Verification items for the finished model (mm, model axes). Round coordinates to 2 decimals unless told otherwise and drop trailing zeros. Write each loop counter-clockwise with the first axis right and the second up, starting at its lowest first coordinate (ties: lowest second). Pieces come first, ordered by that corner, then holes. Notation, with made-up numbers: M -3,8 L 54,8 A17 ccw 54,33 Z; hole C 26.5,22.5 d7. An arc over 180 degrees is marked long. One line per item, written item: value. Start each with the question number.
Item 1: Section check B-B, the plane x = -10. Record the cut outline in (y, z), then the cut area to 3 significant figures.
Item 2: Gauge pin test, flat ends, axial feed: pin 1 (4.5 mm diameter, centred on y = 0, z = 7.5, fed in from -X); pin 2 (12 mm diameter, centred on y = -8, z = 19, fed in from +X); pin 3 (10 mm diameter, centred on x = 9.5, z = 19, fed in from -Y); pin 4 (1 mm diameter, centred on x = 5, z = 7, fed in from +Y). Record the tip position at first contact, or that the pin passes through.
Item 3: Section check A-A, the plane y = 0. Record the cut outline in (x, z), then the cut area to 4 significant figures.
Item 4: Thickness scan on probe 1 along X at (y, z) = (0, 3); probe 2 along Y at (x, z) = (-9, 7). Record the ranges inside material, lowest first. Write a range as from..to.
Item 5: Draft check along Z on faces 1 (the face through (3, 0, 32.5)), 2 (the face through (3, 0, 0)), 3 (the face through (7.395, 0.751, 5.115)). Enter one of: +Z half, -Z half, draft (parallel to the pull), parting line (faces both ways), or undercut.
Item 6: Section check D-D, the plane z = 28. Record the cut outline in (x, y).
Item 7: Section check C-C, the plane y = -12. Record the cut outline in (x, z), then the cut area to 3 significant figures.
from build123d import *

# Parameters (mm, degrees)
SKETCH1_R               = 15
SKETCH1_R_2             = 2.5
BOSS_EXTRUDE1_DEPTH     = 32.5
SKETCH2_R               = 2.5
CUT_EXTRUDE1_DEPTH      = 32.5
CUT_EXTRUDE1_DEPTH_BACK = 32.5


with BuildPart() as part:
    # Sketch1 → Boss-Extrude1 (new body)
    with BuildSketch(Plane.XY):
        Circle(SKETCH1_R)
        Circle(SKETCH1_R_2, mode=Mode.SUBTRACT)
    extrude(amount=BOSS_EXTRUDE1_DEPTH)

    # Sketch2 → Cut-Extrude1 (cut, two sides)
    with BuildSketch(Plane(origin=(0, 0, 0), x_dir=(0, 0, -1), z_dir=(1, 0, 0))) as cut_extrude1_sk:
        with Locations((-7.5, 0)):
            Circle(SKETCH2_R)
    extrude(amount=CUT_EXTRUDE1_DEPTH, mode=Mode.SUBTRACT)
    extrude(cut_extrude1_sk.sketch, amount=-CUT_EXTRUDE1_DEPTH_BACK, mode=Mode.SUBTRACT)


solid = part.part
Response values:
1. outline: M -11.18,0 L 11.18,0 L 11.18,32.5 L -11.18,32.5 Z; hole C 0,7.5 d5
1. area: 707 mm2
2. pin 1: passes through
2. pin 2: stops at x = 14.87
2. pin 3: stops at y = -14.31
2. pin 4: stops at y = 14.31
3. outline: M -15,0 L -2.5,0 L -2.5,5 L -15,5 Z; M -15,10 L -2.5,10 L -2.5,32.5 L -15,32.5 Z; M 2.5,0 L 15,0 L 15,5 L 2.5,5 Z; M 2.5,10 L 15,10 L 15,32.5 L 2.5,32.5 Z
3. area: 687.5 mm2
4. probe 1: x = -15..-2.5, 2.5..15
4. probe 2: y = -12..-2.45, 2.45..12
5. face 1: +Z half
5. face 2: -Z half
5. face 3: undercut
6. outline: C 0,0 d30; hole C 0,0 d5
7. outline: M -9,0 L 9,0 L 9,32.5 L -9,32.5 Z
7. area: 585 mm2
